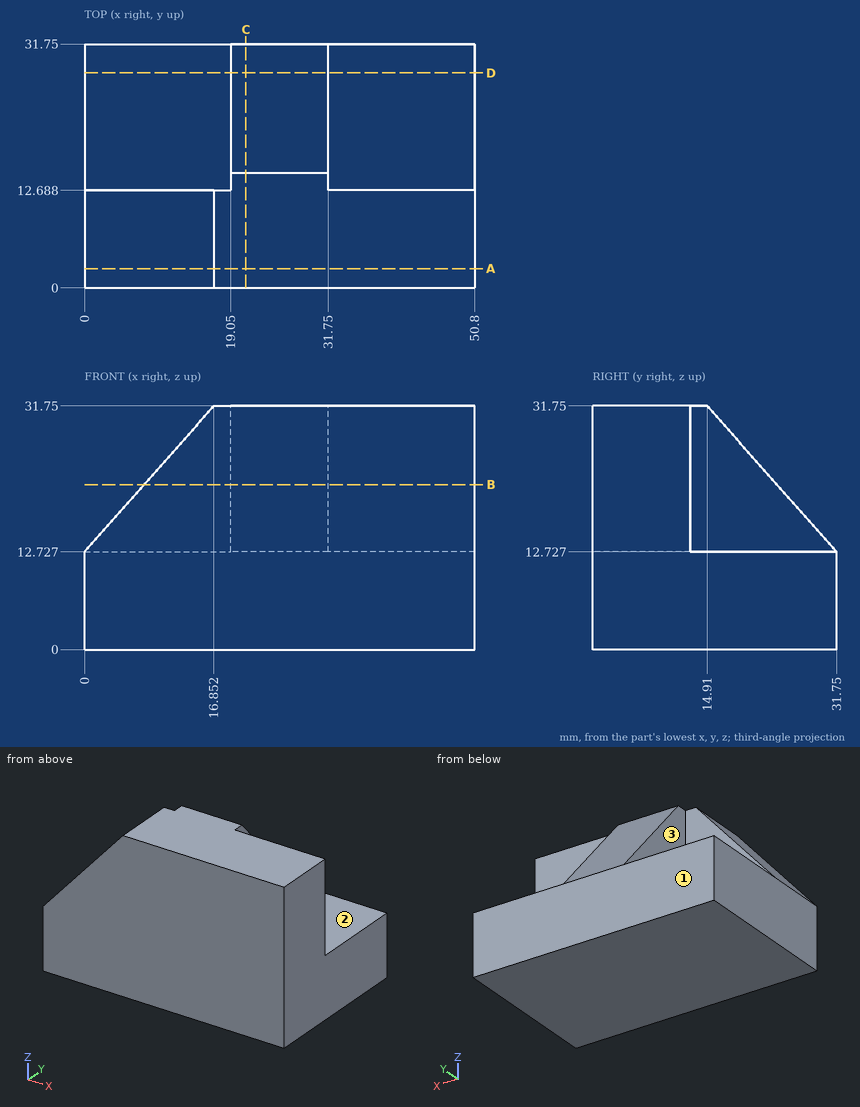
For this review, use the dimensioned drawing (mm, ordinates from the lowest corner) and the shaded views. A direction names the side the tool comes from. Coordinates: 2 decimals unless noted, no trailing zeros. Order: outer loops, then holes, each group sorted by start corner. A loop starts at its lowest first (then second) coordinate and runs counter-clockwise, first axis right, second up. Notation, with made-up numbers: (38, -26) -> (69, -26) arc R30 ccw to (69, 8) -> close; hole circle Ø2 at (9, 40.5). An arc over 180 degrees is marked (long way). One line per item, written item: value. Start each with the question number.
Q1. Take a section at B-B, the plane z = 21.5. State the section outline as (x, y) points, then the cut area to 3 significant figures.
Q2. Take a section at C-C, the plane x = 21. State the section outline as (y, z) points, then the cut area to 3 significant figures.
Q3. Take a section at D-D, the plane y = 28. State the section outline as (x, z) points, then the cut area to 3 significant figures.
Q4. For probe 1 along Y at (x, z) = (41, 20.5); probe 2 along X at (y, z) = (13, 16); probe 3 along Z at (x, y) = (4.5, 18.5), list the stretches that pass through material, from the lowest coordinate up.
Q5. Insertion check: pin 1 Ø15 at (x, z) = (10.5, 27) entering from +Y; pin 2 Ø5.5 at (x, y) = (42.5, 24) entering from +Z; pin 3 Ø6 at (y, z) = (23, 19) entering from +X. Each pin has a flat end and moves straight along its axis. Give the tip position at first contact, or say it passes through.
Q6. Tool access review of the marked faces 1, 2 and 3: name each direction out of +Z, -Z, +X, -X, +Y, -Y from which nothing blocks a thin tool from reaching the whole face with its end or side.
Q7. Take a section at A-A, the plane y = 2.5. State the section outline as (x, z) points.
Values follow:
1. outline: (7.77, 0) -> (50.8, 0) -> (50.8, 12.69) -> (31.75, 12.69) -> (31.75, 23.98) -> (19.05, 23.98) -> (19.05, 12.69) -> (7.77, 12.69) -> close
1. area: 689 mm2
2. outline: (0, 0) -> (31.75, 0) -> (31.75, 12.73) -> (14.91, 31.75) -> (0, 31.75) -> close
2. area: 848 mm2
3. outline: (0, 0) -> (50.8, 0) -> (50.8, 12.73) -> (31.75, 12.73) -> (31.75, 16.96) -> (19.05, 16.96) -> (19.05, 12.73) -> (0, 12.73) -> close
3. area: 700 mm2
4. probe 1: y = 0 to 12.69
4. probe 2: x = 19.05 to 31.75
4. probe 3: z = 0 to 12.73
5. pin 1: stops at y = 12.69
5. pin 2: stops at z = 12.73
5. pin 3: stops at x = 31.75
6. face 1: +Z, -Z, +X, -X, +Y
6. face 2: +Z, +X, +Y
6. face 3: +Z, -X, +Y
7. outline: (0, 0) -> (50.8, 0) -> (50.8, 31.75) -> (16.85, 31.75) -> (0, 12.73) -> close
